Geometry: final body of the model. Coordinates: model frame, mm. Face numbers are marked on the shaded views. Round coordinates to 2 decimals unless told otherwise and drop trailing zeros. Write each loop counter-clockwise with the first axis right and the second up, starting at its lowest first coordinate (ties: lowest second). Pieces come first, ordered by that corner, then holes. Notation, with made-up numbers: M 56.25,5 L 91.25,5 A23 cw 91.25,17 Z; hole C 26,39 d11. An arc over 180 degrees is marked long. Answer as CSV lines item,"result". Start each with the question number.
Q1. First-contact query: pin 1 (5 mm diameter, centred on y = 8.5, z = 21.5, fed in from +X); pin 2 (4 mm diameter, centred on x = 22.5, y = -0.5, fed in from +Z); pin 3 (12 mm diameter, centred on x = -6, z = 19, fed in from -Y). Flat tips, straight axial feed; report the tip coordinate or a pass-through.
Q2. Section query D-D on z = 21. Output: boundary loops of the cut face in (x, y).
Q3. Section query C-C on y = 21.5. Output: boundary loops of the cut face in (x, z), and give its area (3 significant figures).
Q4. Ray query, probe 1 along X at (y, z) = (0, 21.5); probe 2 along Z at (x, y) = (-5.5, 26.6). Return the intervals inside material, ascending.
Q5. Section query B-B on y = 0. Output: boundary loops of the cut face in (x, z).
Q6. Mould query, pull axis X, two halves, no side actions, for the marked faces 1, 2 and 3. Classes: pulls with the +X half, pulls with the -X half, needs draft (parallel to the pull), parting line crosses it, or undercut.
Q7. Section query A-A on x = 0. Output: boundary loops of the cut face in (y, z).
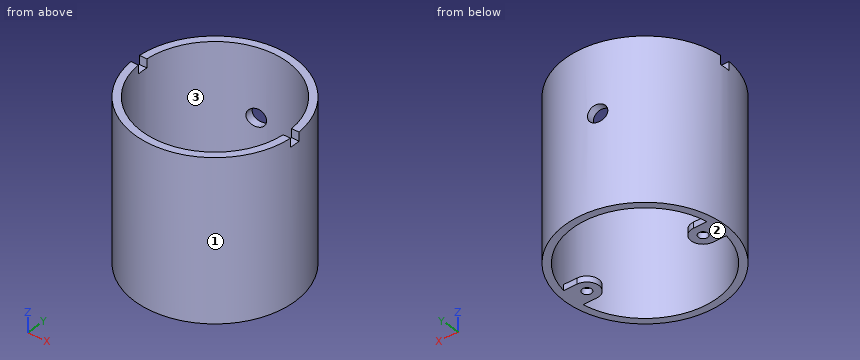
```python
from build123d import *

# Parameters (mm, degrees)
SKETCH1_R           = 27.5
SKETCH1_R_2         = 25
BOSS_EXTRUDE1_DEPTH = 55
SKETCH2_R           = 1.6
BOSS_EXTRUDE2_DEPTH = 2
CUT_EXTRUDE1_START  = 55
SKETCH3_W           = 60.535746445
SKETCH3_H           = 3.6
CUT_EXTRUDE1_DEPTH  = 3
SKETCH4_R           = 3
CUT_EXTRUDE2_DEPTH  = 28.5


with BuildPart() as part:
    # Sketch1 → Boss-Extrude1 (new body)
    with BuildSketch(Plane.XY):
        Circle(SKETCH1_R)
        Circle(SKETCH1_R_2, mode=Mode.SUBTRACT)
    extrude(amount=BOSS_EXTRUDE1_DEPTH)

    # Sketch2 → Boss-Extrude2 (add)
    with BuildSketch(Plane.XY):
        with BuildLine():
            Line((-20, 4.1), (-26.124079623, 4.1))
            Line((-26.124079623, 4.1), (-26.124079623, -4.1))
            Line((-26.124079623, -4.1), (-20, -4.1))
            ThreePointArc((-20, -4.1), (-15.9, 0), (-20, 4.1))
        make_face()
        with Locations((-20, 0)):
            Circle(SKETCH2_R, mode=Mode.SUBTRACT)
        with BuildLine():
            Line((26.124079623, -4.1), (20, -4.1))
            ThreePointArc((20, -4.1), (15.9, 0), (20, 4.1))
            Line((20, 4.1), (26.124079623, 4.1))
            Line((26.124079623, 4.1), (26.124079623, -4.1))
        make_face()
        with Locations((20, 0)):
            Circle(SKETCH2_R, mode=Mode.SUBTRACT)
    extrude(amount=BOSS_EXTRUDE2_DEPTH)

    # Sketch3 → Cut-Extrude1 (cut)
    with BuildSketch(Plane.XY.offset(CUT_EXTRUDE1_START)):
        with Locations((1.235423396, 0)):
            Rectangle(SKETCH3_W, SKETCH3_H)
    extrude(amount=-CUT_EXTRUDE1_DEPTH, mode=Mode.SUBTRACT)

    # Sketch4 → Cut-Extrude2 (cut, through all)
    with BuildSketch(Plane(origin=(0, 0, 0), x_dir=(1, 0, 0), z_dir=(0, 1, 0))):
        with Locations((-5.5, -31.7)):
            Circle(SKETCH4_R)
    extrude(amount=CUT_EXTRUDE2_DEPTH, mode=Mode.SUBTRACT)


solid = part.part
```
Entries:
1,pin 1,"stops at x = 26.84"
1,pin 2,"stops at z = 2"
1,pin 3,"stops at y = -27.5"
2,outline,"C 0,0 d55; hole C 0,0 d50"
3,outline,"M -17.15,0 L -12.76,0 L -12.76,55 L -17.15,55 Z; M 12.76,0 L 17.15,0 L 17.15,55 L 12.76,55 Z"
3,area,"483 mm^2"
4,probe 1,"x = -27.5 to -25, 25 to 27.5"
4,probe 2,"z = 0 to 28.7, 34.7 to 55"
5,outline,"M -27.5,0 L -21.6,0 L -21.6,2 L -25,2 L -25,52 L -27.5,52 Z; M -18.4,0 L -15.9,0 L -15.9,2 L -18.4,2 Z; M 15.9,0 L 18.4,0 L 18.4,2 L 15.9,2 Z; M 21.6,0 L 27.5,0 L 27.5,52 L 25,52 L 25,2 L 21.6,2 Z"
6,face 1,"parting line crosses it"
6,face 2,"needs draft"
6,face 3,"undercut"
7,outline,"M -27.5,0 L -25,0 L -25,55 L -27.5,55 Z; M 25,0 L 27.5,0 L 27.5,55 L 25,55 Z"
